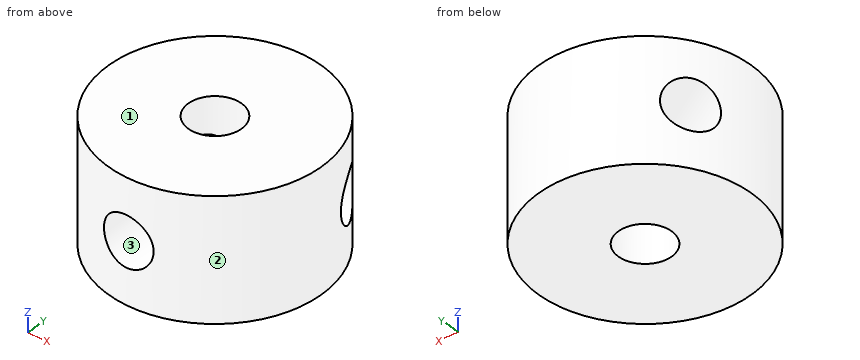
```python
from build123d import *

# Parameters (mm, degrees)
F0_R     = 7
F0_R_2   = 1.75
F1_DEPTH = 4
F2_R     = 1.65
F3_DEPTH = 7
F4_COUNT = 3
F5_DEPTH = 7
F6_DEPTH = 7
F7_DEPTH = 7


with BuildPart() as f1:
    # F0 (on Top) → F1 (new body, symmetric)
    with BuildSketch(Plane.XY):
        Circle(F0_R)
        Circle(F0_R_2, mode=Mode.SUBTRACT)
    extrude(amount=F1_DEPTH, both=True)


with BuildPart() as f3:
    # F2 (on Front) → F3 (new body)
    with BuildSketch(Plane.XZ):
        Circle(F2_R)
    extrude(amount=F3_DEPTH)


with BuildPart() as f4_1:
    # F4: instance of F3
    add(f3.part.rotate(Axis((0, 0, 4), (0, 0, 1)), 1 * 360 / F4_COUNT))


with BuildPart() as f4_2:
    # F4: instance of F3
    add(f3.part.rotate(Axis((0, 0, 4), (0, 0, 1)), 2 * 360 / F4_COUNT))


with BuildPart() as f5_tool:
    # F5 (cut): a face of the model
    f5_faces = [f3.part.faces().sort_by_distance(p)[0] for p in [
        (0, -7, 0),
    ]]
    extrude(f5_faces, amount=-F5_DEPTH)


with BuildPart() as f1_1:
    add(f1.part)

    # F5: cut by f5_tool
    add(f5_tool.part, mode=Mode.SUBTRACT)


with BuildPart() as f3_1:
    add(f3.part)

    # F5: cut by f5_tool
    add(f5_tool.part, mode=Mode.SUBTRACT)


with BuildPart() as f4_1_1:
    add(f4_1.part)

    # F5: cut by f5_tool
    add(f5_tool.part, mode=Mode.SUBTRACT)


with BuildPart() as f4_2_1:
    add(f4_2.part)

    # F5: cut by f5_tool
    add(f5_tool.part, mode=Mode.SUBTRACT)


with BuildPart() as f6_tool:
    # F6 (cut): a face of the model
    f6_faces = [f4_1_1.part.faces().sort_by_distance(p)[0] for p in [
        (6.0621778265, 3.5, 0),
    ]]
    extrude(f6_faces, amount=-F6_DEPTH)


with BuildPart() as f1_2:
    add(f1_1.part)

    # F6: cut by f6_tool
    add(f6_tool.part, mode=Mode.SUBTRACT)


with BuildPart() as f4_1_2:
    add(f4_1_1.part)

    # F6: cut by f6_tool
    add(f6_tool.part, mode=Mode.SUBTRACT)


with BuildPart() as f4_2_2:
    add(f4_2_1.part)

    # F6: cut by f6_tool
    add(f6_tool.part, mode=Mode.SUBTRACT)


with BuildPart() as f7_tool:
    # F7 (cut): a face of the model
    f7_faces = [f4_2_2.part.faces().sort_by_distance(p)[0] for p in [
        (-6.0621778265, 3.5, 0),
    ]]
    extrude(f7_faces, amount=-F7_DEPTH)


with BuildPart() as f1_3:
    add(f1_2.part)

    # F7: cut by f7_tool
    add(f7_tool.part, mode=Mode.SUBTRACT)


with BuildPart() as f4_2_3:
    add(f4_2_2.part)

    # F7: cut by f7_tool
    add(f7_tool.part, mode=Mode.SUBTRACT)


solid = f1_3.part
```
For this review, take the finished solid that the model builds, in its own axes (mm). Face numbers are marked on the shaded views. Coordinates: 2 decimals unless noted, no trailing zeros. Write each loop counter-clockwise with the first axis right and the second up, starting at its lowest first coordinate (ties: lowest second). Pieces come first, ordered by that corner, then holes. Notation, with made-up numbers: (23, 74) - (58, 74) arc R11 cw to (58, 95) - close; hole circle Ø3 at (48.25, -22.5). An arc over 180 degrees is marked (long way). Answer in a Markdown table with one row per item. Add a question column.
Q1. Draft analysis for pull direction X (two halves, no side actions). For the marked faces 1, 2 and 3, state which applies: +X half, -X half, draft (parallel to the pull), parting line (faces both ways), or undercut.
Q2. We need section A-A, the plane z = 0. State the section outline as (x, y) points.
Q3. We need section C-C, the plane x = -0.75. Count the separate pieces of the cut face and the enclosed holes in it, and give its area (3 significant figures).
Q4. For probe 1 along Y at (x, z) = (0, 2.65); probe 2 along Z at (x, y) = (0, -4.75); probe 3 along Y at (x, z) = (1, 2.25), list the stretches that pass through material, from the lowest coordinate up.
Q5. We need section B-B, the plane y = -4.25. State the section outline as (x, z) points, and give its area (3 significant figures).
Q6. For P1, Ø3, axis at x = -4.5, z = 0.5, coming from the +Y side, flat-tipped, find the tip position at first contact; note if it passes through.
Answer list:
| question | item | result |
|---|---|---|
| 1 | face 1 | draft |
| 1 | face 2 | parting line |
| 1 | face 3 | undercut |
| 2 | outline | (-6.72, 1.97) arc R7 ccw to (-1.65, -6.8) - (-1.65, -0.95) - close; (-5.07, 4.83) - (0, 1.91) - (5.07, 4.83) arc R7 ccw to start; (1.65, -6.8) arc R7 ccw to (6.72, 1.97) - (1.65, -0.95) - close |
| 3 | separate pieces | 3 |
| 3 | enclosed holes | 0 |
| 3 | area | 68.9 mm2 |
| 4 | probe 1 | y = -7 to -1.75, 1.75 to 7 |
| 4 | probe 2 | z = -4 to -1.65, 1.65 to 4 |
| 4 | probe 3 | y = -6.93 to -1.44, 1.44 to 6.93 |
| 5 | outline | (-5.56, -4) - (5.56, -4) - (5.56, 4) - (-5.56, 4) - close; hole circle Ø3.3 at (0, 0) |
| 5 | area | 80.4 mm2 |
| 6 | P1 | stops at y = 6.32 |
